Autodesk Inventor part; units mm, degrees
ref_plane "YZ Plane" through (0, 0, 0) normal (1, 0, 0) x (0, 1, 0)
ref_plane "XZ Plane" through (0, 0, 0) normal (0, 1, 0) x (-1, 0, 0)
ref_plane "XY Plane" through (0, 0, 0) normal (0, 0, 1) x (1, 0, 0)
sketch "Sketch1" plane through (0, 0, 0) normal (0, 0, 1) x (1, 0, 0)
  line L0 (0, 0) -> (160, 0)
  line L1 (160, 0) -> (160, 160)
  line L2 (160, 160) -> (0, 160)
  line L3 (0, 160) -> (0, 0)
  dimension "d0" = 160
  dimension "d1" = 160
extrude "Extrusion1" add sketch "Sketch1" along normal blind 10
sketch "Sketch2" plane through (0, 0, 10) normal (0, 0, 1) x (1, 0, 0)
  line L0 (0, 0) -> (160, 0)
  line L1 (0, 0) -> (10, 0)
  line L2 (10, 0) -> (10, 150)
  line L3 (10, 150) -> (150, 150)
  dimension "d4" = 10
  dimension "d5" = 150
  dimension "d6" = 140
sketch "Sketch3" plane through (0, 0, 10) normal (0, 0, 1) x (1, 0, 0)
  line L0 (150.8125, 150.8125) -> (150.8125, 10.8125)
  line L1 (150.8125, 10.8125) -> (10.8125, 10.8125)
  line L2 (10.8125, 10.8125) -> (10.8125, 80.8125)
  line L3 (10.8125, 80.8125) -> (150.8125, 80.8125)
  circle A0 centre (10.8125, 150.8125) radius 5
  circle A1 centre (150.8125, 150.8125) radius 5
  circle A2 centre (150.8125, 10.8125) radius 5
  circle A3 centre (10.8125, 10.8125) radius 5
  point P0 (0, 0)
  dimension "d7" = 140
  dimension "d8" = 140
  dimension "d9" = 70
  dimension "d10" = 140
  dimension "d11" = 10
  dimension "d12" = 10
  dimension "d14" = 10
  dimension "d15" = 10
extrude "Extrusion2" [suppressed]
sketch "Sketch4" plane through (0, 0, 10) normal (0, 0, 1) x (1, 0, 0)
  line L0 (0, 160) -> (0, 0)
  line L1 (0, 80) -> (30, 80)
  line L2 (30, 80) -> (33, 80)
  line L3 (33, 80) -> (36.5125, 80)
  line L4 (36.5125, 80) -> (41.275, 80)
  circle A0 centre (38.8938, 80) radius 8.5
  dimension "d19" = 30
  dimension "d36" = 3
  dimension "d40" = 17
extrude "Extrusion3" cut sketch "Sketch4" against normal through all
sketch "Sketch5" plane through (0, 0, 10) normal (0, 0, 1) x (1, 0, 0)
  line L0 (0, 160.3375) -> (9.9943, 160)
  line L1 (160, 160) -> (0, 160)
  line L2 (9.9943, 160) -> (159.9943, 160)
  line L3 (159.9943, 160) -> (159.9943, 0)
  line L4 (159.9943, 0) -> (147.6375, 0)
  point P0 (0, 0)
  dimension "d23" = 10
  dimension "d24" = 150
sketch "Sketch6" plane through (0, 0, 10) normal (0, 0, 1) x (1, 0, 0)
  line L0 (160, 160) -> (0, 160)
  line L1 (160, 160) -> (160, 150)
  line L2 (160, 0) -> (160, 160)
  line L3 (160, 150) -> (10, 150)
  line L4 (10, 150) -> (10, 10)
  line L5 (0, 0) -> (160, 0)
  dimension "d25" = 10
  dimension "d26" = 150
  dimension "d27" = 140
sketch "Sketch7" plane through (0, 0, 10) normal (0, 0, 1) x (1, 0, 0)
  line L0 (9.525, 9.525) -> (149.525, 9.525)
  line L1 (149.525, 9.525) -> (149.525, 149.525)
  circle A0 centre (9.525, 9.525) radius 5
  circle A1 centre (9.525, 149.525) radius 5
  circle A2 centre (149.525, 149.525) radius 5
  circle A3 centre (149.525, 9.525) radius 5
  point P0 (0, 0)
  dimension "d28" = 140
  dimension "d29" = 140
  dimension "d30" = 10
  dimension "d31" = 10
  dimension "d32" = 10
  dimension "d33" = 10
extrude "Extrusion4" cut sketch "Sketch7" against normal through all
properties part number "2 nd part of capping syStem"
Geometry check sheet. Reference: the model listing, model coordinates, mm. Coordinates: 2 decimals unless noted, no trailing zeros. Order: outer loops, then holes, each group sorted by start corner. A loop starts at its lowest first (then second) coordinate and runs counter-clockwise, first axis right, second up. Notation, with made-up numbers: (76.25, 43) - (128.25, 43) arc R29 ccw to (128.25, 69) - close; hole circle Ø10 at (23.25, -28). An arc over 180 degrees is marked (long way). Answer in a Markdown table with one row per item. Add a question column.
1. Gauge pin test, flat ends, axial feed: pin 1 Ø22 at (x, y) = (38.89, 80) entering from +Z; pin 2 Ø6 at (x, y) = (149.525, 9.525) entering from -Z. Record the tip position at first contact, or that the pin passes through.
2. Draft check along Y on faces 1 (the face through (81, 160, 5)), 2 (the face through (148.441, 144.644, 5.07)), 3 (the face through (32.148, 74.828, 5.07)), 4 (the face through (0, 81, 5)). Enter one of: +Y half, -Y half, draft (parallel to the pull), parting line (faces both ways), or undercut.
3. Section check B-B (z = 8.25). Enter the section's corners in (x, y) (3 decimals), plus the area to 3 significant figures.
4. Section check A-A (y = 80). Enter the section's corners in (x, z), plus the area to 3 significant figures.
5. Material ranges on L1, parallel to X at y = 80, z = 6; L2, parallel to X at y = 12.5, z = 7.25; L3, parallel to X at y = 148, z = 4.5, recorded low to high. Write a range as [from, to].
Data:
| question | item | result |
|---|---|---|
| 1 | pin 1 | stops at z = 10 |
| 1 | pin 2 | passes through |
| 2 | face 1 | +Y half |
| 2 | face 2 | undercut |
| 2 | face 3 | undercut |
| 2 | face 4 | draft |
| 3 | outline | (0, 0) - (160, 0) - (160, 160) - (0, 160) - close; hole circle Ø10 at (9.525, 9.525); hole circle Ø10 at (9.525, 149.525); hole circle Ø17 at (38.894, 80); hole circle Ø10 at (149.525, 9.525); hole circle Ø10 at (149.525, 149.525) |
| 3 | area | 25,100 mm² |
| 4 | outline | (0, 0) - (30.39, 0) - (30.39, 10) - (0, 10) - close; (47.39, 0) - (160, 0) - (160, 10) - (47.39, 10) - close |
| 4 | area | 1,430 mm² |
| 5 | L1 | x = [0, 30.39], [47.39, 160] |
| 5 | L2 | x = [0, 5.51], [13.54, 145.51], [153.54, 160] |
| 5 | L3 | x = [0, 4.76], [14.29, 144.76], [154.29, 160] |
